Model file for the job. Use its own axes, mm. A direction names the side the tool comes from. Round coordinates to 2 decimals unless told otherwise and drop trailing zeros. Write each loop counter-clockwise with the first axis right and the second up, starting at its lowest first coordinate (ties: lowest second). Pieces come first, ordered by that corner, then holes.
```python
from build123d import *

# Parameters (mm, degrees)
SKETCH_1_W          = 44.2
SKETCH_1_H          = 20
EXTRUDE_1_DEPTH     = 2
CUT_EXTRUDE_1_REACH = 26.339
SKETCH_2_R          = 3
SKETCH_2_R_2        = 1.65
SKETCH_3_W          = 20
SKETCH_3_H          = 25
EXTRUDE_2_DEPTH     = 2
CUT_EXTRUDE_2_REACH = 54.751
SKETCH_4_R          = 1
CUT_EXTRUDE_3_REACH = 54.751
SKETCH_5_R          = 4
SKETCH_5_R_2        = 1


with BuildPart() as part:
    # 草图1 → 凸台-拉伸1 (new body)
    with BuildSketch(Plane(origin=(0, 0, 0), x_dir=(1, 0, 0), z_dir=(0, 1, 0))):
        Rectangle(SKETCH_1_W, SKETCH_1_H)
    extrude(amount=EXTRUDE_1_DEPTH)

    # 草图2 → 切除-拉伸1 (cut, up to next)
    with BuildSketch(Plane(origin=(0, 2, 0), x_dir=(1, 0, 0), z_dir=(0, 1, 0)), mode=Mode.PRIVATE) as cut_extrude_1_sk1:
        with Locations(Location((0, 0, 0), (0, 0, 270))):
            Circle(SKETCH_2_R)
    cut_extrude_1_tool1 = extrude(cut_extrude_1_sk1.sketch, amount=-CUT_EXTRUDE_1_REACH, mode=Mode.PRIVATE) & part.part
    # 草图2 → 切除-拉伸1 (cut, up to next)
    with BuildSketch(Plane(origin=(0, 2, 0), x_dir=(1, 0, 0), z_dir=(0, 1, 0)), mode=Mode.PRIVATE) as cut_extrude_1_sk2:
        with Locations(Location((0, 7, 0), (0, 0, 270))):
            Circle(SKETCH_2_R_2)
    cut_extrude_1_tool2 = extrude(cut_extrude_1_sk2.sketch, amount=-CUT_EXTRUDE_1_REACH, mode=Mode.PRIVATE) & part.part
    # 草图2 → 切除-拉伸1 (cut, up to next)
    with BuildSketch(Plane(origin=(0, 2, 0), x_dir=(1, 0, 0), z_dir=(0, 1, 0)), mode=Mode.PRIVATE) as cut_extrude_1_sk3:
        with Locations(Location((7, 0, 0), (0, 0, 270))):
            Circle(SKETCH_2_R_2)
    cut_extrude_1_tool3 = extrude(cut_extrude_1_sk3.sketch, amount=-CUT_EXTRUDE_1_REACH, mode=Mode.PRIVATE) & part.part
    # 草图2 → 切除-拉伸1 (cut, up to next)
    with BuildSketch(Plane(origin=(0, 2, 0), x_dir=(1, 0, 0), z_dir=(0, 1, 0)), mode=Mode.PRIVATE) as cut_extrude_1_sk4:
        with Locations(Location((0, -7, 0), (0, 0, 270))):
            Circle(SKETCH_2_R_2)
    cut_extrude_1_tool4 = extrude(cut_extrude_1_sk4.sketch, amount=-CUT_EXTRUDE_1_REACH, mode=Mode.PRIVATE) & part.part
    # 草图2 → 切除-拉伸1 (cut, up to next)
    with BuildSketch(Plane(origin=(0, 2, 0), x_dir=(1, 0, 0), z_dir=(0, 1, 0)), mode=Mode.PRIVATE) as cut_extrude_1_sk5:
        with Locations(Location((-7, 0, 0), (0, 0, 270))):
            Circle(SKETCH_2_R_2)
    cut_extrude_1_tool5 = extrude(cut_extrude_1_sk5.sketch, amount=-CUT_EXTRUDE_1_REACH, mode=Mode.PRIVATE) & part.part
    add(cut_extrude_1_tool1.solids().sort_by_distance((0, 2, 0))[0], mode=Mode.SUBTRACT)
    add(cut_extrude_1_tool2.solids().sort_by_distance((0, 2, -7))[0], mode=Mode.SUBTRACT)
    add(cut_extrude_1_tool3.solids().sort_by_distance((7, 2, 0))[0], mode=Mode.SUBTRACT)
    add(cut_extrude_1_tool4.solids().sort_by_distance((0, 2, 7))[0], mode=Mode.SUBTRACT)
    add(cut_extrude_1_tool5.solids().sort_by_distance((-7, 2, 0))[0], mode=Mode.SUBTRACT)

    # 草图3 → 凸台-拉伸2 (add)
    with BuildSketch(Plane.ZY.offset(22.1)):
        with Locations((0, 14.5)):
            Rectangle(SKETCH_3_W, SKETCH_3_H)
    extrude_2 = extrude(amount=-EXTRUDE_2_DEPTH)

    # 镜向2: 凸台-拉伸2 across plane
    add(extrude_2.mirror(Plane.ZY))

    # 草图4 → 切除-拉伸2 (cut, up to next)
    with BuildSketch(Plane.ZY.offset(22.1), mode=Mode.PRIVATE) as cut_extrude_2_sk1:
        with BuildLine():
            ThreePointArc((-10, 17), (-7.071067812, 24.071067812), (0, 27))
            Line((0, 27), (-10, 27))
            Line((-10, 27), (-10, 17))
        make_face()
    cut_extrude_2_tool1 = extrude(cut_extrude_2_sk1.sketch, amount=-CUT_EXTRUDE_2_REACH, mode=Mode.PRIVATE) & part.part
    # 草图4 → 切除-拉伸2 (cut, up to next)
    with BuildSketch(Plane.ZY.offset(22.1), mode=Mode.PRIVATE) as cut_extrude_2_sk2:
        with BuildLine():
            Line((10, 27), (0, 27))
            ThreePointArc((0, 27), (7.071067812, 24.071067812), (10, 17))
            Line((10, 17), (10, 27))
        make_face()
    cut_extrude_2_tool2 = extrude(cut_extrude_2_sk2.sketch, amount=-CUT_EXTRUDE_2_REACH, mode=Mode.PRIVATE) & part.part
    # 草图4 → 切除-拉伸2 (cut, up to next)
    with BuildSketch(Plane.ZY.offset(22.1), mode=Mode.PRIVATE) as cut_extrude_2_sk3:
        with BuildLine():
            ThreePointArc((1, 10), (0.707106781, 10.707106781), (0, 11))
            Line((0, 11), (0, 9))
            ThreePointArc((0, 9), (0.707106781, 9.292893219), (1, 10))
        make_face()
    cut_extrude_2_tool3 = extrude(cut_extrude_2_sk3.sketch, amount=-CUT_EXTRUDE_2_REACH, mode=Mode.PRIVATE) & part.part
    # 草图4 → 切除-拉伸2 (cut, up to next)
    with BuildSketch(Plane.ZY.offset(22.1), mode=Mode.PRIVATE) as cut_extrude_2_sk4:
        with BuildLine():
            Line((0, 9), (0, 11))
            ThreePointArc((0, 11), (-1, 10), (0, 9))
        make_face()
    cut_extrude_2_tool4 = extrude(cut_extrude_2_sk4.sketch, amount=-CUT_EXTRUDE_2_REACH, mode=Mode.PRIVATE) & part.part
    # 草图4 → 切除-拉伸2 (cut, up to next)
    with BuildSketch(Plane.ZY.offset(22.1), mode=Mode.PRIVATE) as cut_extrude_2_sk5:
        with BuildLine():
            ThreePointArc((1, 10), (0.707106781, 10.707106781), (0, 11))
            Line((0, 11), (0, 9))
            ThreePointArc((0, 9), (0.707106781, 9.292893219), (1, 10))
        make_face()
    cut_extrude_2_tool5 = extrude(cut_extrude_2_sk5.sketch, amount=-CUT_EXTRUDE_2_REACH, mode=Mode.PRIVATE) & part.part
    # 草图4 → 切除-拉伸2 (cut, up to next)
    with BuildSketch(Plane.ZY.offset(22.1), mode=Mode.PRIVATE) as cut_extrude_2_sk6:
        with BuildLine():
            Line((0, 9), (0, 11))
            ThreePointArc((0, 11), (-1, 10), (0, 9))
        make_face()
    cut_extrude_2_tool6 = extrude(cut_extrude_2_sk6.sketch, amount=-CUT_EXTRUDE_2_REACH, mode=Mode.PRIVATE) & part.part
    # 草图4 → 切除-拉伸2 (cut, up to next)
    with BuildSketch(Plane.ZY.offset(22.1), mode=Mode.PRIVATE) as cut_extrude_2_sk7:
        with BuildLine():
            ThreePointArc((4, 17), (2.828427125, 19.828427125), (0, 21))
            Line((0, 21), (0, 13))
            ThreePointArc((0, 13), (2.828427125, 14.171572875), (4, 17))
        make_face()
    cut_extrude_2_tool7 = extrude(cut_extrude_2_sk7.sketch, amount=-CUT_EXTRUDE_2_REACH, mode=Mode.PRIVATE) & part.part
    # 草图4 → 切除-拉伸2 (cut, up to next)
    with BuildSketch(Plane.ZY.offset(22.1), mode=Mode.PRIVATE) as cut_extrude_2_sk8:
        with BuildLine():
            Line((0, 13), (0, 21))
            ThreePointArc((0, 21), (-4, 17), (0, 13))
        make_face()
    cut_extrude_2_tool8 = extrude(cut_extrude_2_sk8.sketch, amount=-CUT_EXTRUDE_2_REACH, mode=Mode.PRIVATE) & part.part
    # 草图4 → 切除-拉伸2 (cut, up to next)
    with BuildSketch(Plane.ZY.offset(22.1), mode=Mode.PRIVATE) as cut_extrude_2_sk9:
        with BuildLine():
            ThreePointArc((4, 17), (2.828427125, 19.828427125), (0, 21))
            Line((0, 21), (0, 13))
            ThreePointArc((0, 13), (2.828427125, 14.171572875), (4, 17))
        make_face()
    cut_extrude_2_tool9 = extrude(cut_extrude_2_sk9.sketch, amount=-CUT_EXTRUDE_2_REACH, mode=Mode.PRIVATE) & part.part
    # 草图4 → 切除-拉伸2 (cut, up to next)
    with BuildSketch(Plane.ZY.offset(22.1), mode=Mode.PRIVATE) as cut_extrude_2_sk10:
        with BuildLine():
            Line((0, 13), (0, 21))
            ThreePointArc((0, 21), (-4, 17), (0, 13))
        make_face()
    cut_extrude_2_tool10 = extrude(cut_extrude_2_sk10.sketch, amount=-CUT_EXTRUDE_2_REACH, mode=Mode.PRIVATE) & part.part
    # 草图4 → 切除-拉伸2 (cut, up to next)
    with BuildSketch(Plane.ZY.offset(22.1), mode=Mode.PRIVATE) as cut_extrude_2_sk11:
        with Locations((7, 17)):
            Circle(SKETCH_4_R)
    cut_extrude_2_tool11 = extrude(cut_extrude_2_sk11.sketch, amount=-CUT_EXTRUDE_2_REACH, mode=Mode.PRIVATE) & part.part
    # 草图4 → 切除-拉伸2 (cut, up to next)
    with BuildSketch(Plane.ZY.offset(22.1), mode=Mode.PRIVATE) as cut_extrude_2_sk12:
        with Locations((0, 24)):
            Circle(SKETCH_4_R)
    cut_extrude_2_tool12 = extrude(cut_extrude_2_sk12.sketch, amount=-CUT_EXTRUDE_2_REACH, mode=Mode.PRIVATE) & part.part
    # 草图4 → 切除-拉伸2 (cut, up to next)
    with BuildSketch(Plane.ZY.offset(22.1), mode=Mode.PRIVATE) as cut_extrude_2_sk13:
        with Locations((-7, 17)):
            Circle(SKETCH_4_R)
    cut_extrude_2_tool13 = extrude(cut_extrude_2_sk13.sketch, amount=-CUT_EXTRUDE_2_REACH, mode=Mode.PRIVATE) & part.part
    add(cut_extrude_2_tool1.solids().sort_by_distance((-22.1, 24.766321, -7.766321))[0], mode=Mode.SUBTRACT)
    add(cut_extrude_2_tool2.solids().sort_by_distance((-22.1, 24.766321, 7.766321))[0], mode=Mode.SUBTRACT)
    add(cut_extrude_2_tool3.solids().sort_by_distance((-22.1, 10, 0.424413))[0], mode=Mode.SUBTRACT)
    add(cut_extrude_2_tool4.solids().sort_by_distance((-22.1, 10, -0.424413))[0], mode=Mode.SUBTRACT)
    add(cut_extrude_2_tool5.solids().sort_by_distance((-22.1, 10, 0.424413))[0], mode=Mode.SUBTRACT)
    add(cut_extrude_2_tool6.solids().sort_by_distance((-22.1, 10, -0.424413))[0], mode=Mode.SUBTRACT)
    add(cut_extrude_2_tool7.solids().sort_by_distance((-22.1, 17, 1.697653))[0], mode=Mode.SUBTRACT)
    add(cut_extrude_2_tool8.solids().sort_by_distance((-22.1, 17, -1.697653))[0], mode=Mode.SUBTRACT)
    add(cut_extrude_2_tool9.solids().sort_by_distance((-22.1, 17, 1.697653))[0], mode=Mode.SUBTRACT)
    add(cut_extrude_2_tool10.solids().sort_by_distance((-22.1, 17, -1.697653))[0], mode=Mode.SUBTRACT)
    add(cut_extrude_2_tool11.solids().sort_by_distance((-22.1, 17, 7))[0], mode=Mode.SUBTRACT)
    add(cut_extrude_2_tool12.solids().sort_by_distance((-22.1, 24, 0))[0], mode=Mode.SUBTRACT)
    add(cut_extrude_2_tool13.solids().sort_by_distance((-22.1, 17, -7))[0], mode=Mode.SUBTRACT)

    # 草图5 → 切除-拉伸3 (cut, up to next)
    with BuildSketch(Plane(origin=(22.1, 0, 0), x_dir=(0, 0, -1), z_dir=(1, 0, 0)), mode=Mode.PRIVATE) as cut_extrude_3_sk1:
        with Locations(Location((0, 17, 0), (0, 0, 180))):
            Circle(SKETCH_5_R)
    cut_extrude_3_tool1 = extrude(cut_extrude_3_sk1.sketch, amount=-CUT_EXTRUDE_3_REACH, mode=Mode.PRIVATE) & part.part
    # 草图5 → 切除-拉伸3 (cut, up to next)
    with BuildSketch(Plane(origin=(22.1, 0, 0), x_dir=(0, 0, -1), z_dir=(1, 0, 0)), mode=Mode.PRIVATE) as cut_extrude_3_sk2:
        with Locations((-7.5, 24.5)):
            Circle(SKETCH_5_R_2)
    cut_extrude_3_tool2 = extrude(cut_extrude_3_sk2.sketch, amount=-CUT_EXTRUDE_3_REACH, mode=Mode.PRIVATE) & part.part
    # 草图5 → 切除-拉伸3 (cut, up to next)
    with BuildSketch(Plane(origin=(22.1, 0, 0), x_dir=(0, 0, -1), z_dir=(1, 0, 0)), mode=Mode.PRIVATE) as cut_extrude_3_sk3:
        with Locations((7.5, 24.5)):
            Circle(SKETCH_5_R_2)
    cut_extrude_3_tool3 = extrude(cut_extrude_3_sk3.sketch, amount=-CUT_EXTRUDE_3_REACH, mode=Mode.PRIVATE) & part.part
    # 草图5 → 切除-拉伸3 (cut, up to next)
    with BuildSketch(Plane(origin=(22.1, 0, 0), x_dir=(0, 0, -1), z_dir=(1, 0, 0)), mode=Mode.PRIVATE) as cut_extrude_3_sk4:
        with Locations((7.5, 9.5)):
            Circle(SKETCH_5_R_2)
    cut_extrude_3_tool4 = extrude(cut_extrude_3_sk4.sketch, amount=-CUT_EXTRUDE_3_REACH, mode=Mode.PRIVATE) & part.part
    # 草图5 → 切除-拉伸3 (cut, up to next)
    with BuildSketch(Plane(origin=(22.1, 0, 0), x_dir=(0, 0, -1), z_dir=(1, 0, 0)), mode=Mode.PRIVATE) as cut_extrude_3_sk5:
        with Locations((-7.5, 9.5)):
            Circle(SKETCH_5_R_2)
    cut_extrude_3_tool5 = extrude(cut_extrude_3_sk5.sketch, amount=-CUT_EXTRUDE_3_REACH, mode=Mode.PRIVATE) & part.part
    add(cut_extrude_3_tool1.solids().sort_by_distance((22.1, 17, 0))[0], mode=Mode.SUBTRACT)
    add(cut_extrude_3_tool2.solids().sort_by_distance((22.1, 24.5, 7.5))[0], mode=Mode.SUBTRACT)
    add(cut_extrude_3_tool3.solids().sort_by_distance((22.1, 24.5, -7.5))[0], mode=Mode.SUBTRACT)
    add(cut_extrude_3_tool4.solids().sort_by_distance((22.1, 9.5, -7.5))[0], mode=Mode.SUBTRACT)
    add(cut_extrude_3_tool5.solids().sort_by_distance((22.1, 9.5, 7.5))[0], mode=Mode.SUBTRACT)


solid = part.part
```
1) Flat gauge pins, fed straight in: pin 1 Ø2 at (x, z) = (7, 0) entering from +Y; pin 2 Ø4 at (x, z) = (-7.5, 6.5) entering from +Y; pin 3 Ø1.8 at (y, z) = (9.5, -7.5) entering from +X. Where does each tip first touch, or does it go through?
2) Pull direction Z, two halves, no side cores. Call faces 1 (the face through (2, 1, 10)), 2 (the face through (-20.1, 12, 0)), 3 (the face through (-8, 1.01, -1.31)): released by +Z, released by -Z, zero draft, split by the parting line, or undercut.
3) Cut at D-D on x = -7. List the corners of the cut face in (y, z), and give its area (3 significant figures).
4) Cut at C-C on z = 3.5. List the corners of the cut face in (x, y).
5) Cut at A-A on x = 0. List the corners of the cut face in (y, z), and give its area (3 significant figures).
6) Cut at B-B on z = -7.5. List the corners of the cut face in (x, y).
7) Wall check: probe 1 along Y at (x, z) = (20.8, 7.5); probe 2 along X at (y, z) = (5, 4.25); probe 3 along Z at (x, y) = (21.45, 17). Give the ranges that are in metal, low to high.
8) Which spindle directions (+Z, -Z, +X, -X, +Y, -Y) get a long thin tool onto all of the face, cutting with end or side? Do faces 4 (the face through (0, 2, -5)), 5 (the face through (21.114, 23.524, -7.283)), 6 (the face through (-21, 16, 7)), 7 (the face through (2, 1, -10)), 8 (the face through (5.4, 1, -0.4)). Say none if no direction does.
Result sheet:
1. pin 1: passes through
1. pin 2: stops at y = 2
1. pin 3: stops at x = -20.1
2. face 1: released by +Z
2. face 2: zero draft
2. face 3: undercut
3. outline: (0, -10) - (2, -10) - (2, -1.65) - (0, -1.65) - close; (0, 1.65) - (2, 1.65) - (2, 10) - (0, 10) - close
3. area: 33.4 mm2
4. outline: (-22.1, 0) - (22.1, 0) - (22.1, 15.06) - (20.1, 15.06) - (20.1, 2) - (-20.1, 2) - (-20.1, 15.06) - (-22.1, 15.06) - close; (-22.1, 18.94) - (-20.1, 18.94) - (-20.1, 26.37) - (-22.1, 26.37) - close; (20.1, 18.94) - (22.1, 18.94) - (22.1, 27) - (20.1, 27) - close
5. outline: (0, -10) - (2, -10) - (2, -8.65) - (0, -8.65) - close; (0, -5.35) - (2, -5.35) - (2, -3) - (0, -3) - close; (0, 3) - (2, 3) - (2, 5.35) - (0, 5.35) - close; (0, 8.65) - (2, 8.65) - (2, 10) - (0, 10) - close
5. area: 14.8 mm2
6. outline: (-22.1, 0) - (-1.57, 0) - (-1.57, 2) - (-20.1, 2) - (-20.1, 16.13) - (-22.1, 16.13) - close; (-22.1, 17.87) - (-20.1, 17.87) - (-20.1, 23.61) - (-22.1, 23.61) - close; (1.57, 0) - (22.1, 0) - (22.1, 8.5) - (20.1, 8.5) - (20.1, 2) - (1.57, 2) - close; (20.1, 10.5) - (22.1, 10.5) - (22.1, 23.5) - (20.1, 23.5) - close; (20.1, 25.5) - (22.1, 25.5) - (22.1, 27) - (20.1, 27) - close
7. probe 1: y = 0 to 8.5, 10.5 to 23.5, 25.5 to 27
7. probe 2: x = -22.1 to -20.1, 20.1 to 22.1
7. probe 3: z = -10 to -4, 4 to 10
8. face 4: +Z, -Z, +Y
8. face 5: +X
8. face 6: -X
8. face 7: -Z, +X, -X, +Y, -Y
8. face 8: +Y, -Y
